Design review of the part shown in the three views and the two pictorial views. Dimensions are in mm from the part's minimum x, y and z. A direction names the side the tool comes from. Round coordinates to 2 decimals unless told otherwise and drop trailing zeros. Order: outer loops, then holes, each group sorted by start corner. A loop starts at its lowest first (then second) coordinate and runs counter-clockwise, first axis right, second up. Notation, with made-up numbers: M 42.25,-7.5 L 88.25,-7.5 A10 ccw 88.25,-3.5 Z; hole C 40.5,26 d8. An arc over 180 degrees is marked long. Write each question's results on one line, items separated by ' | '. Start each with the question number.
Item 1: Wall thickness on line 1 (Y direction, x = 22.5, z = 2.15); line 2 (Y direction, x = 3.5, z = 8.05); line 3 (X direction, y = 12.75, z = 7.5): over which ranges is each line inside the solid? List them lowest first. Write a range as [from, to].
Item 2: Machinability: for the marked faces 4, 5, 6, 7 and 8, which of the approach directions +Z, -Z, +X, -X, +Y, -Y give a long, thin tool a straight path to every point of the face, cutting with its end or side? Answer none if there is none.
Item 3: The part is to be moulded in two halves that separate along Y. For the marked faces 1, 2 and 3, say which applies: +Y half, -Y half, draft (parallel to the pull), parting line (faces both ways), or undercut.
Item 4: Take a section at D-D, the plane z = 7.25. Write out the cut boundary in (x, y).
Item 5: Clearance check with flat-ended pins moving along their axes: pin 1 (1.4 mm diameter, centred on x = 22.5, y = 13.5, fed in from +Z); pin 2 (4.5 mm diameter, centred on x = 3.5, y = 13.5, fed in from -Z); pin 3 (1.9 mm diameter, centred on x = 22.5, y = 21, fed in from +Z); pin 4 (3 mm diameter, centred on x = 17.5, z = 6.5, fed in from -Y). State where each tip first meets the part, or that it passes through.
Item 6: Take a section at A-A, the plane x = 3.5. Write out the cut boundary in (y, z).
Item 7: Take a section at B-B, the plane y = 4. Write out the cut boundary in (x, z).
Item 8: Take a section at C-C, the plane x = 22.5. Write out the cut boundary in (y, z), plus the area to 3 significant figures.
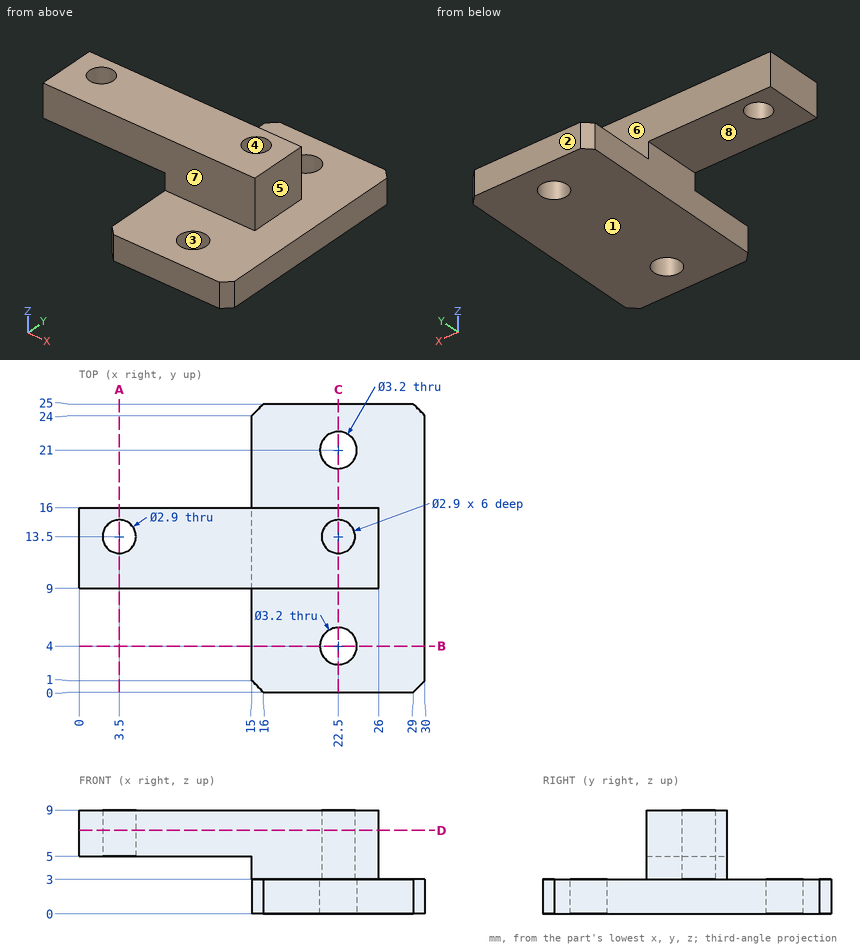
Results list:
1) line 1: [0, 2.4], [5.6, 19.4], [22.6, 25] | line 2: [9, 12.05], [14.95, 16] | line 3: [0, 2.26], [4.74, 21.26], [23.74, 26]
2) face 4: +Z | face 5: +Z, +X, +Y, -Y | face 6: +Z, +X, -X, +Y | face 7: +Z, +X, -X, -Y | face 8: -Z, -X, +Y, -Y
3) face 1: draft | face 2: +Y half | face 3: undercut
4) outline: M 0,9 L 26,9 L 26,16 L 0,16 Z; hole C 3.5,13.5 d2.9; hole C 22.5,13.5 d2.9
5) pin 1: z = 3 | pin 2: z = 5 | pin 3: through | pin 4: y = 9
6) outline: M 9,5 L 12.05,5 L 12.05,9 L 9,9 Z; M 14.95,5 L 16,5 L 16,9 L 14.95,9 Z
7) outline: M 15,0 L 20.9,0 L 20.9,3 L 15,3 Z; M 24.1,0 L 30,0 L 30,3 L 24.1,3 Z
8) outline: M 0,0 L 2.4,0 L 2.4,3 L 0,3 Z; M 5.6,0 L 19.4,0 L 19.4,3 L 16,3 L 16,9 L 14.95,9 L 14.95,3 L 12.05,3 L 12.05,9 L 9,9 L 9,3 L 5.6,3 Z; M 22.6,0 L 25,0 L 25,3 L 22.6,3 Z | area: 80.4 mm²
